Autodesk Inventor part; units mm, degrees
ref_plane "YZ Plane" through (0, 0, 0) normal (1, 0, 0) x (0, 1, 0)
ref_plane "XZ Plane" through (0, 0, 0) normal (0, 1, 0) x (-1, 0, 0)
ref_plane "XY Plane" through (0, 0, 0) normal (0, 0, 1) x (1, 0, 0)
sketch "스케치1" plane through (0, 0, 0) normal (0, 1, 0) x (-1, 0, 0)
  line L0 (-10.9012, 33.5504) -> (10.9012, 33.5504)
  line L1 (10.9012, 33.5504) -> (28.5397, 20.7353)
  line L2 (28.5397, 20.7353) -> (35.277, 0)
  line L3 (35.277, 0) -> (28.5397, -20.7353)
  line L4 (28.5397, -20.7353) -> (10.9012, -33.5504)
  line L5 (10.9012, -33.5504) -> (-10.9012, -33.5504)
  line L6 (-10.9012, -33.5504) -> (-28.5397, -20.7353)
  line L7 (-28.5397, -20.7353) -> (-35.277, 0)
  line L8 (-35.277, 0) -> (-28.5397, 20.7353)
  line L9 (-28.5397, 20.7353) -> (-10.9012, 33.5504)
  line L10 (11.9409, -36.7504) -> (-11.9409, -36.7504)
  line L11 (-11.9409, -36.7504) -> (-31.2618, -22.713)
  line L12 (-31.2618, -22.713) -> (-38.6417, 0)
  line L13 (-38.6417, 0) -> (-31.2618, 22.713)
  line L14 (-31.2618, 22.713) -> (-11.9409, 36.7504)
  line L15 (-11.9409, 36.7504) -> (11.9409, 36.7504)
  line L16 (11.9409, 36.7504) -> (31.2618, 22.713)
  line L17 (31.2618, 22.713) -> (38.6417, 0)
  line L18 (38.6417, 0) -> (31.2618, -22.713)
  line L19 (31.2618, -22.713) -> (11.9409, -36.7504)
  point P0 (0, 0)
  point P1 (0, 0)
  point P2 (0, 0)
  dimension "d0" = 70.554
  dimension "d1" = 3.2
extrude "돌출1" add sketch "스케치1" along normal blind 4.4 contours L0 L1 L2 L3 L4 L5 L6 L7 L8 L9 | L10 L11 L12 L13 L14 L15 L16 L17 L18 L19
sketch "스케치2" plane through (0, 4.4, 0) normal (0, 1, 0) x (1, 0, 0)
  line L0 (-11.4211, 35.1504) -> (11.4211, 35.1504)
  line L1 (11.4211, 35.1504) -> (29.9007, 21.7242)
  line L2 (29.9007, 21.7242) -> (36.9593, 0)
  line L3 (36.9593, 0) -> (29.9007, -21.7242)
  line L4 (29.9007, -21.7242) -> (11.4211, -35.1504)
  line L5 (11.4211, -35.1504) -> (-11.4211, -35.1504)
  line L6 (-11.4211, -35.1504) -> (-29.9007, -21.7242)
  line L7 (-29.9007, -21.7242) -> (-36.9593, 0)
  line L8 (-36.9593, 0) -> (-29.9007, 21.7242)
  line L9 (-29.9007, 21.7242) -> (-11.4211, 35.1504)
  line L10 (-31.2618, 22.713) -> (-38.6417, 0)
  point P0 (0, 0)
  point P1 (0, 0)
  dimension "d4" = 1.6
extrude "돌출2" cut sketch "스케치2" against normal blind 1.2
sketch "스케치3" plane through (0, 3.2, 0) normal (0, 1, 0) x (1, 0, 0)
  line L0 (-10.7712, 33.1504) -> (10.7712, 33.1504)
  line L1 (10.7712, 33.1504) -> (28.1994, 20.4881)
  line L2 (28.1994, 20.4881) -> (34.8564, 0)
  line L3 (34.8564, 0) -> (28.1994, -20.4881)
  line L4 (28.1994, -20.4881) -> (10.7712, -33.1504)
  line L5 (10.7712, -33.1504) -> (-10.7712, -33.1504)
  line L6 (-10.7712, -33.1504) -> (-28.1994, -20.4881)
  line L7 (-28.1994, -20.4881) -> (-34.8564, 0)
  line L8 (-34.8564, 0) -> (-28.1994, 20.4881)
  line L9 (-28.1994, 20.4881) -> (-10.7712, 33.1504)
  line L10 (-29.9007, 21.7242) -> (-11.4211, 35.1504)
  point P0 (0, 0)
  point P1 (0, 0)
  dimension "d7" = 2
extrude "돌출3" add sketch "스케치3" along normal blind 0.6
fillet "모깎기1" radius 1.2 20 edges at (0, 4.4, 36.7504) (0, 0, 36.7504) (-21.6014, 4.4, 29.7317) (-21.6014, 0, 29.7317) (-34.9517, 4.4, 11.3565) (-34.9517, 4.4, -11.3565) (-21.6014, 4.4, -29.7317) (0, 4.4, -36.7504) (21.6014, 4.4, -29.7317) (34.9517, 4.4, -11.3565) (34.9517, 4.4, 11.3565) (21.6014, 4.4, 29.7317) (21.6014, 0, -29.7317) (0, 0, -36.7504) (-21.6014, 0, -29.7317) (-34.9517, 0, -11.3565) (-34.9517, 0, 11.3565) (34.9517, 0, -11.3565) (34.9517, 0, 11.3565) (21.6014, 0, 29.7317)
sketch "스케치4" plane through (0, 0, 0) normal (0, -1, 0) x (1, 0, 0)
  line L0 (-7.5, -10) -> (-2.5, -10)
  line L1 (-2.5, -10) -> (-2.5, 10)
  line L2 (-2.5, 10) -> (-7.5, 10)
  line L3 (-7.5, 10) -> (-7.5, -10)
  line L4 (-7.5, -10) -> (-2.5, 10) construction
  line L5 (-2.5, -10) -> (-7.5, 10) construction
  line L6 (7.5, -10) -> (2.5, -10)
  line L7 (2.5, -10) -> (2.5, 10)
  line L8 (2.5, 10) -> (7.5, 10)
  line L9 (7.5, 10) -> (7.5, -10)
  line L10 (7.5, -10) -> (2.5, 10) construction
  line L11 (2.5, -10) -> (7.5, 10) construction
  point P0 (0, 0)
  point P1 (-5, 0)
  point P2 (5, 0)
  dimension "d11" = 5
  dimension "d12" = 20
  dimension "d13" = 5
  dimension "d14" = 20
  dimension "d15" = 5
  dimension "d16" = 2.5
extrude "돌출4" add sketch "스케치4" along normal blind 10
sketch "스케치5" plane through (-7.5, 0, -10) normal (-1, 0, 0) x (0, 0, 1)
  circle A0 centre (15, -5) radius 1.25
  circle A1 centre (5, -5) radius 1.25
  line L0 (0, 0) -> (0, -10)
  line L1 (-11.9714, 0) -> (10, 0)
  dimension "d19" = 2.5
  dimension "d20" = 2.5
  dimension "d21" = 5
  dimension "d22" = 5
  dimension "d23" = 10
extrude "돌출5" cut sketch "스케치5" against normal up to surface (15 mm away)
properties part number "OV-PAM_n_10_bottom"
Read the model definition and answer for the solid it produces. Units are mm, in the model's axes. A direction names the side the tool comes from. Coordinates: 2 decimals unless noted, no trailing zeros. Write each loop counter-clockwise with the first axis right and the second up, starting at its lowest first coordinate (ties: lowest second). Pieces come first, ordered by that corner, then holes. Notation, with made-up numbers: (1.5, 54.5) -> (60.5, 54.5) arc R24 ccw to (60.5, 72.5) -> close; hole circle Ø9 at (12, -11.75). An arc over 180 degrees is marked (long way). Write item = value, one per line.
(1) For a pull along Z with two mould halves and no side action, classify faces 4 (the face through (0, 2, -36.75)), 5 (the face through (1, 0, 0)), 6 (the face through (4.96, -6.22, 4.73)) as +Z half, -Z half, draft (parallel to the pull), parting line (faces both ways), or undercut.
From the geometry:
face_4 = -Z half
face_5 = draft
face_6 = undercut
(2) Given pin 1 Ø4 at (y, z) = (1, -16.5) entering from +X; pin 2 Ø3 at (y, z) = (1, 12) entering from +X; pin 3 Ø2 at (y, z) = (-5, 5) entering from -X; pin 4 Ø3 at (y, z) = (-5, -5) entering from +X, each flat-ended and moving along its own axis, determine where each tip first touches the part or whether it passes through.
From the geometry:
pin_1 = 33.93
pin_2 = 35.23
pin_3 = through
pin_4 = 7.5
(3) Straight lines are drawn through the part: L1, parallel to Y at x = -4, z = 5; L2, parallel to X at y = -8.75, z = -0.5; L3, parallel to Y at x = -6, z = 19. For each, find the intervals that lie inside material, in ascending order. Write a range as from..to.
From the geometry:
L1 = -10..-6.25, -3.75..3.8
L2 = -7.5..-2.5, 2.5..7.5
L3 = 0..3.8
(4) Section C-C on z = -5 is taken. Count the separate pieces of the cut face and the enclosed holes in it, plus the area to 3 significant figures.
From the geometry:
separate_pieces = 3
enclosed_holes = 0
area = 355 mm2
(5) Section B-B on x = 1.5 is taken. Write down the section's boundary in (y, z), plus the area to 3 significant figures.
From the geometry:
outline = (0, -35.55) arc R1.2 ccw to (1.2, -36.75) -> (3.2, -36.75) arc R1.2 ccw to (4.4, -35.55) -> (4.4, -35.15) -> (3.2, -35.15) -> (3.2, -33.15) -> (3.8, -33.15) -> (3.8, 33.15) -> (3.2, 33.15) -> (3.2, 35.15) -> (4.4, 35.15) -> (4.4, 35.55) arc R1.2 ccw to (3.2, 36.75) -> (1.2, 36.75) arc R1.2 ccw to (0, 35.55) -> close
area = 278 mm2
(6) Which of the six approach directions +Z, -Z, +X, -X, +Y, -Y give full straight-line access (tool end or side, diameter ignored) to faces 1 (the face through (5, -5, -10)), 2 (the face through (5, -5, 10)), 3 (the face through (-19.61, 3.5, -26.73))?
From the geometry:
face_1 = -Z, +X, -X, -Y
face_2 = +Z, +X, -X, -Y
face_3 = +Y
(7) Section A-A on y = -7.25 is taken. Write down the section's boundary in (x, z), plus the area to 3 significant figures.
From the geometry:
outline = (-7.5, -10) -> (-2.5, -10) -> (-2.5, 10) -> (-7.5, 10) -> close; (2.5, -10) -> (7.5, -10) -> (7.5, 10) -> (2.5, 10) -> close
area = 200 mm2
